Model file for the job. Use its own axes, mm. A direction names the side the tool comes from. Give positions to 0.01 mm unless a question says otherwise; leave off trailing zeros. Loops run counter-clockwise (first coordinate to the right, second up) from the corner with the lowest first, then second, coordinate; pieces in that order, holes last. Notation, with made-up numbers: M 69.5,86.25 L 125.5,86.25 A12 cw 125.5,96.25 Z; hole C -5,80.5 d7. An arc over 180 degrees is marked long. Use CSV: the item, a comma, the result in double quotes. Start each with the question number.
(1) Slice it at A-A on x = 10. List the corners of the cut face in (y, z) (3 decimals).
(2) Two-plate mould, pull along Y, no slides. Class faces 1 (the face through (22.66, 2.75, 11.11)), 2 (the face through (45.212, -15, 0)): pulls with the +Y half, pulls with the -Y half, needs draft (parallel to the pull), parting line crosses it, or undercut.
(3) Wall check: line 1 along Z through (x, y) = (52.5, -14.5); line 2 along Z through (x, y) = (37.5, -21); line 3 along X through (y, z) = (19, 6). Give the ranges that are in metal, low to high. Write a range as from..to.
(4) Slice it at B-B on x = 63.5. List the corners of the cut face in (y, z).
(5) Flat gauge pins, fed straight in: P1, Ø0.8, axis at x = 16, y = 11, coming from the +Z side; P2, Ø3.5, axis at y = -14, z = 0.5, coming from the +X side; P3, Ø1.3, axis at x = 12, y = 11.5, coming from the -Z side. Where does each tip first touch, or does it go through?
(6) Tool access for faces 3 (the face through (61.66, 0.35, -19.77)), 4 (the face through (59, 0, -14.294)), 5 (the face through (22, -11, -3.175)): list every direction of +Z, -Z, +X, -X, +Y, -Y with a clear straight run to the whole face (end or side of a thin tool).
```python
from build123d import *

# Parameters (mm, degrees)
SKETCH1_R           = 25.4
BOSS_EXTRUDE1_DEPTH = 83.08975
CUT_EXTRUDE1_DEPTH  = 43.688
SKETCH5_R           = 7.94258
CUT_EXTRUDE2_DEPTH  = 43.688
SKETCH6_W           = 13.49375
SKETCH6_H           = 14.29385
CUT_EXTRUDE3_DEPTH  = 43.688
CHAMFER1_SIZE       = 1.524
SKETCH8_R           = 10.16
CUT_EXTRUDE4_DEPTH  = 91.521967399
CUT_EXTRUDE5_DEPTH  = 91.521967399
CIRPATTERN1_COUNT   = 6


with BuildPart() as part:
    # Sketch1 → Boss-Extrude1 (new body)
    with BuildSketch(Plane(origin=(0, 0, 0), x_dir=(0, 0, -1), z_dir=(1, 0, 0))):
        Circle(SKETCH1_R)
    extrude(amount=BOSS_EXTRUDE1_DEPTH)

    # Sketch4 → Cut-Extrude1 (cut, symmetric)
    with BuildSketch(Plane.XY):
        with BuildLine():
            ThreePointArc((69.596, 13.49375), (79.137522129, 9.541522129), (83.08975, 0))
            Line((83.08975, 0), (83.08975, 25.4))
            Line((83.08975, 25.4), (36.9170127, 25.4))
            ThreePointArc((36.9170127, 25.4), (52.205808799, 16.563033999), (69.596, 13.49375))
        make_face()
        with BuildLine():
            Line((36.9170127, -25.4), (83.08975, -25.4))
            Line((83.08975, -25.4), (83.08975, 0))
            ThreePointArc((83.08975, 0), (79.137522129, -9.541522129), (69.596, -13.49375))
            ThreePointArc((69.596, -13.49375), (52.205808799, -16.563033999), (36.9170127, -25.4))
        make_face()
    extrude(amount=CUT_EXTRUDE1_DEPTH, both=True, mode=Mode.SUBTRACT)

    # Sketch5 → Cut-Extrude2 (cut, symmetric)
    with BuildSketch(Plane.XY):
        with Locations((69.596, 0)):
            Circle(SKETCH5_R)
    extrude(amount=CUT_EXTRUDE2_DEPTH, both=True, mode=Mode.SUBTRACT)

    # Sketch6 → Cut-Extrude3 (cut, symmetric)
    with BuildSketch(Plane(origin=(0, 0, 0), x_dir=(1, 0, 0), z_dir=(0, 1, 0))):
        with BuildLine():
            Line((69.596, 0), (69.596, 14.29385))
            Line((69.596, 14.29385), (49.784, 14.29385))
            ThreePointArc((49.784, 14.29385), (46.551107796, 12.954742204), (45.212, 9.72185))
            Line((45.212, 9.72185), (45.212, 0))
            Line((45.212, 0), (69.596, 0))
        make_face()
        with BuildLine():
            Line((69.596, -14.29385), (69.596, 0))
            Line((69.596, 0), (45.212, 0))
            Line((45.212, 0), (45.212, -9.72185))
            ThreePointArc((45.212, -9.72185), (46.551107796, -12.954742204), (49.784, -14.29385))
            Line((49.784, -14.29385), (69.596, -14.29385))
        make_face()
        with Locations((76.342875, -7.146925)):
            Rectangle(SKETCH6_W, SKETCH6_H)
        with Locations((76.342875, 7.146925)):
            Rectangle(SKETCH6_W, SKETCH6_H)
    extrude(amount=CUT_EXTRUDE3_DEPTH, both=True, mode=Mode.SUBTRACT)

    # Chamfer1
    chamfer1_edges = [part.edges().sort_by_distance(p)[0] for p in [
        (0, 0, 25.4),
    ]]
    chamfer(chamfer1_edges, length=CHAMFER1_SIZE)

    # Sketch8 → Cut-Extrude4 (cut, through all)
    with BuildSketch(Plane.ZY):
        Circle(SKETCH8_R)
    extrude(amount=-CUT_EXTRUDE4_DEPTH, mode=Mode.SUBTRACT)

    # Sketch7 → Cut-Extrude5 (cut, through all)
    with BuildSketch(Plane.ZY):
        with BuildLine():
            Line((-3.175, 9.651164438), (-3.175, 12.296722124))
            ThreePointArc((-3.175, 12.296722124), (0, 12.7), (3.175, 12.296722124))
            Line((3.175, 12.296722124), (3.175, 9.651164438))
            ThreePointArc((3.175, 9.651164438), (0, 10.16), (-3.175, 9.651164438))
        make_face()
    cut_extrude5 = extrude(amount=-CUT_EXTRUDE5_DEPTH, mode=Mode.SUBTRACT)

    # CirPattern1: Cut-Extrude5 ×6 about axis
    cirpattern1_axis = Axis((0, 0, 0), (1, 0, 0))
    for i in range(1, CIRPATTERN1_COUNT):
        add(cut_extrude5.rotate(cirpattern1_axis, i * 360 / CIRPATTERN1_COUNT), mode=Mode.SUBTRACT)


solid = part.part
```
Reply:
1,outline,"C 0,0 d50.8; hole M -12.297,-3.175 L -9.651,-3.175 A10.16 ccw -7.575,-6.771 L -8.898,-9.062 A12.7 ccw -3.399,-12.237 L -2.076,-9.946 A10.16 ccw 2.076,-9.946 L 3.399,-12.237 A12.7 ccw 8.898,-9.062 L 7.575,-6.771 A10.16 ccw 9.651,-3.175 L 12.297,-3.175 A12.7 ccw 12.297,3.175 L 9.651,3.175 A10.16 ccw 7.575,6.771 L 8.898,9.062 A12.7 ccw 3.399,12.237 L 2.076,9.946 A10.16 ccw -2.076,9.946 L -3.399,12.237 A12.7 ccw -8.898,9.062 L -7.575,6.771 A10.16 ccw -9.651,3.175 L -12.297,3.175 A12.7 ccw Z"
2,face 1,"undercut"
2,face 2,"needs draft"
3,line 1,"z = -20.85..-14.29, 14.29..20.85"
3,line 2,"z = -14.29..14.29"
3,line 3,"x = 0..45.21"
4,outline,"M -13.86,-21.28 A25.4 ccw -5.09,-24.88 L -5.09,-14.29 L -13.86,-14.29 Z; M -13.86,14.29 L -5.09,14.29 L -5.09,24.88 A25.4 ccw -13.86,21.28 Z; M 5.09,-24.88 A25.4 ccw 13.86,-21.28 L 13.86,-14.29 L 5.09,-14.29 Z; M 5.09,14.29 L 13.86,14.29 L 13.86,21.28 A25.4 ccw 5.09,24.88 Z"
5,P1,"stops at z = 23.08"
5,P2,"stops at x = 45.21"
5,P3,"stops at z = -22.97"
6,face 3,"+Z, -Z"
6,face 4,"+X, +Y, -Y"
6,face 5,"+X, -X"
